Source: CAD feature listing. Evaluate the final solid. Frame: model axes, mm. A direction names the side the tool comes from. Give positions to 0.01 mm unless a question says otherwise; leave off trailing zeros. Loops run counter-clockwise (first coordinate to the right, second up) from the corner with the lowest first, then second, coordinate; pieces in that order, holes last.
from build123d import *

# Parameters (mm, degrees)
F0_R     = 28.575
F1_DEPTH = 25.4


with BuildPart() as f1:
    # F0 (on Front) → F1 (new body)
    with BuildSketch(Plane.XZ):
        with BuildLine():
            ThreePointArc((-69.669226, 32.890535), (-79.327388, 35.337363), (-88.9, 38.1))
            ThreePointArc((-88.9, 38.1), (-127, 0), (-88.9, -38.1))
            ThreePointArc((-88.9, -38.1), (-79.484753, -35.438589), (-69.9901, -33.076059))
            ThreePointArc((-69.9901, -33.076059), (-55.9449, -19.119922), (-50.8, 0))
            ThreePointArc((-50.8, 0), (-55.852288, 18.959397), (-69.669226, 32.890535))
        make_face()
        with Locations((-88.9, 0)):
            Circle(F0_R, mode=Mode.SUBTRACT)
        with BuildLine():
            ThreePointArc((-69.669226, 32.890535), (-78.938057, 36.77458), (-88.9, 38.1))
            ThreePointArc((-88.9, 38.1), (-79.327388, 35.337363), (-69.669226, 32.890535))
        make_face()
        with BuildLine():
            ThreePointArc((-69.9901, -33.076059), (-79.484753, -35.438589), (-88.9, -38.1))
            ThreePointArc((-88.9, -38.1), (-79.117052, -36.822601), (-69.9901, -33.076059))
        make_face()
        with BuildLine():
            ThreePointArc((69.669226, 32.890535), (0, 24.782982), (-69.669226, 32.890535))
            ThreePointArc((-69.669226, 32.890535), (-55.852288, 18.959397), (-50.8, 0))
            ThreePointArc((-50.8, 0), (-55.9449, -19.119922), (-69.9901, -33.076059))
            ThreePointArc((-69.9901, -33.076059), (0, -25.059942), (69.9901, -33.076059))
            ThreePointArc((69.9901, -33.076059), (50.800451, -0.185323), (69.669226, 32.890535))
        make_face()
        with BuildLine():
            ThreePointArc((88.9, 38.1), (79.327388, 35.337363), (69.669226, 32.890535))
            ThreePointArc((69.669226, 32.890535), (50.800451, -0.185323), (69.9901, -33.076059))
            ThreePointArc((69.9901, -33.076059), (79.484753, -35.438589), (88.9, -38.1))
            ThreePointArc((88.9, -38.1), (115.840768, -26.940768), (127, 0))
            ThreePointArc((127, 0), (115.840768, 26.940768), (88.9, 38.1))
        make_face()
        with Locations((88.9, 0)):
            Circle(F0_R, mode=Mode.SUBTRACT)
        with BuildLine():
            ThreePointArc((88.9, 38.1), (78.938057, 36.77458), (69.669226, 32.890535))
            ThreePointArc((69.669226, 32.890535), (79.327388, 35.337363), (88.9, 38.1))
        make_face()
        with BuildLine():
            ThreePointArc((88.9, -38.1), (79.484753, -35.438589), (69.9901, -33.076059))
            ThreePointArc((69.9901, -33.076059), (79.117052, -36.822601), (88.9, -38.1))
        make_face()
    extrude(amount=F1_DEPTH)


solid = f1.part
1) Cut plane B-B (y = -14). Return loops of the section in (x, z) (3 decimals).
Checks:
outline: (-88.9, -38.1) arc R38.1 ccw to (-69.99, -33.076) arc R309.556 cw to (69.99, -33.076) arc R38.1 ccw to (88.9, -38.1) arc R38.1 ccw to (127, 0) arc R38.1 ccw to (88.9, 38.1) arc R38.1 ccw to (69.669, 32.891) arc R303.392 cw to (-69.669, 32.891) arc R38.1 ccw to (-88.9, 38.1) arc R38.1 ccw to start; hole circle Ø57.15 at (-88.9, 0); hole circle Ø57.15 at (88.9, 0)
2) Pull-direction query (X, two-part tool) for faces 1 (the flat face through (-2, 0, 1)), 2 (the cylindrical face through (-0.99, -12.52, -25.06)); classes: released by +X, released by -X, zero draft, split by the parting line, or undercut.
Checks:
face 1: zero draft
face 2: undercut
3) Cut plane A-A (z = 21). Return loops of the section in (x, y), and give its area (3 significant figures).
Checks:
outline: (-120.69, -25.4) - (-108.28, -25.4) - (-108.28, 0) - (-120.69, 0) - close; (-69.52, -25.4) - (69.52, -25.4) - (69.52, 0) - (-69.52, 0) - close; (108.28, -25.4) - (120.69, -25.4) - (120.69, 0) - (108.28, 0) - close
area: 4,160 mm2
4) Reachability of faces 3 (the cylindrical face through (-117.447, -12.522, 1.256)), 4 (the cylindrical face through (79.07, -12.52, 36.81)) from +Z, -Z, +X, -X, +Y, -Y: full face, straight path, thin tool, end or side. Return the list, or none.
Checks:
face 3: +Y, -Y
face 4: +Z, +Y, -Y
5) Cut plane C-C (x = 102.5). Return loops of the section in (y, z).
Checks:
outline: (-25.4, -35.59) - (0, -35.59) - (0, -25.13) - (-25.4, -25.13) - close; (-25.4, 25.13) - (0, 25.13) - (0, 35.59) - (-25.4, 35.59) - close
6) Contact query for flat-ended pins moving along their axis: P1, Ø4, axis at y = -13, z = 11.5, coming from the -X side; P2, Ø10, axis at x = -24.5, y = -19, coming from the +Z side; P3, Ø4, axis at y = -13.5, z = -19, coming from the -X side. Output: stop coordinate, or through.
Checks:
P1: stops at x = -125.8
P2: stops at z = 26.22
P3: stops at x = -123
7) Ray query, probe 1 along Z at (x, y) = (-88.9, -8.25) (3 decimals); probe 2 along X at (y, z) = (-22.75, 15.5); probe 3 along X at (y, z) = (-15, 7). Return the intervals inside material, ascending.
Checks:
probe 1: z = -38.1 to -28.575, 28.575 to 38.1
probe 2: x = -123.7 to -112.91, -64.89 to 64.89, 112.91 to 123.7
probe 3: x = -126.35 to -116.6, -61.2 to 61.2, 116.6 to 126.35
8) Cut plane D-D (z = -17). Return loops of the section in (x, y), and give its area (3 significant figures).
Checks:
outline: (-123, -25.4) - (-111.87, -25.4) - (-111.87, 0) - (-123, 0) - close; (-65.93, -25.4) - (65.93, -25.4) - (65.93, 0) - (-65.93, 0) - close; (111.87, -25.4) - (123, -25.4) - (123, 0) - (111.87, 0) - close
area: 3,910 mm2
